Input: part model. Units: mm. Frame: model coordinates. Face numbers are marked on the shaded views. A direction names the side the tool comes from. Coordinates: 2 decimals unless noted, no trailing zeros. Loops run counter-clockwise (first coordinate to the right, second up) from the corner with the lowest first, then second, coordinate; pieces in that order, holes last.
```python
from build123d import *

# Parameters (mm, degrees)
CROQUIS1_W              = 30
CROQUIS1_H              = 30
SALIENTE_EXTRUIR1_DEPTH = 3
CROQUIS2_W              = 3
CROQUIS2_H              = 30
SALIENTE_EXTRUIR2_DEPTH = 30
REDONDEO1_R             = 15
CROQUIS3_R              = 4
CORTAR_EXTRUIR1_DEPTH   = 48.053161424
CROQUIS4_R              = 3
CORTAR_EXTRUIR2_DEPTH   = 37.742346142
CHAFL_N1_SIZE           = 2


with BuildPart() as part:
    # Croquis1 → Saliente-Extruir1 (new body)
    with BuildSketch(Plane(origin=(0, 0, 0), x_dir=(1, 0, 0), z_dir=(0, 1, 0))):
        Rectangle(CROQUIS1_W, CROQUIS1_H)
    extrude(amount=SALIENTE_EXTRUIR1_DEPTH)

    # Croquis2 → Saliente-Extruir2 (add)
    with BuildSketch(Plane(origin=(0, 3, 0), x_dir=(1, 0, 0), z_dir=(0, 1, 0))):
        with Locations((-13.5, 0)):
            Rectangle(CROQUIS2_W, CROQUIS2_H)
        with Locations((13.5, 0)):
            Rectangle(CROQUIS2_W, CROQUIS2_H)
    extrude(amount=SALIENTE_EXTRUIR2_DEPTH)

    # Redondeo1
    redondeo1_edges = [part.edges().sort_by_distance(p)[0] for p in [
        (-13.5, 33, -15),
        (13.5, 33, -15),
        (13.5, 33, 15),
        (-13.5, 33, 15),
    ]]
    fillet(redondeo1_edges, radius=REDONDEO1_R - 0.0001)  # a hair under: the kernel refuses the full size

    # Croquis3 → Cortar-Extruir1 (cut, through all)
    with BuildSketch(Plane(origin=(15, 0, 0), x_dir=(0, 0, -1), z_dir=(1, 0, 0))):
        with Locations((0, 18)):
            Circle(CROQUIS3_R)
    extrude(amount=-CORTAR_EXTRUIR1_DEPTH, mode=Mode.SUBTRACT)

    # Croquis4 → Cortar-Extruir2 (cut, through all)
    with BuildSketch(Plane(origin=(0, 3, 0), x_dir=(1, 0, 0), z_dir=(0, 1, 0))):
        with Locations(Location((0, 0, 0), (0, 0, 270))):
            Circle(CROQUIS4_R)
    extrude(amount=-CORTAR_EXTRUIR2_DEPTH, mode=Mode.SUBTRACT)

    # Chaflán1
    chafl_n1_edges = [part.edges().sort_by_distance(p)[0] for p in [
        (0, 3, -3),
    ]]
    chamfer(chafl_n1_edges, length=CHAFL_N1_SIZE)


solid = part.part
```
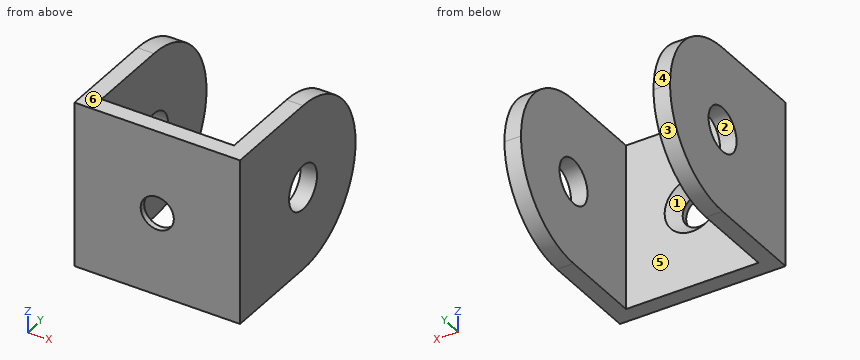
Item 1: Section query B-B (y = 12.5). Output: boundary loops of the cut face in (x, z), then the cut area to 3 significant figures.
Result:
outline: (-15, -15) - (-12, -15) - (-12, 15) - (-15, 15) - close; (12, -15) - (15, -15) - (15, 15) - (12, 15) - close
area: 180 mm2
Item 2: Mould query, pull axis Z, two halves, no side actions, for the marked faces 1, 2, 3 and 4. Classes: +Z half, -Z half, draft (parallel to the pull), parting line (faces both ways), or undercut.
Result:
face 1: undercut
face 2: undercut
face 3: -Z half
face 4: +Z half
Item 3: Section query A-A (x = 0). Output: boundary loops of the cut face in (y, z), then the cut area to 3 significant figures.
Result:
outline: (0, -15) - (3, -15) - (3, -5) - (1, -3) - (0, -3) - close; (0, 3) - (1, 3) - (3, 5) - (3, 15) - (0, 15) - close
area: 68.0 mm2
Item 4: Section query D-D (y = 24.5). Output: boundary loops of the cut face in (x, z).
Result:
outline: (-15, -13.52) - (-12, -13.52) - (-12, 13.52) - (-15, 13.52) - close; (12, -13.52) - (15, -13.52) - (15, 13.52) - (12, 13.52) - close
Item 5: Line query: L1, parallel to Y at x = -14.25, z = 0; L2, parallel to X at y = 23.5, z = -11; L3, parallel to X at y = 0.25, z = 0. Output: solid intervals per line, ascending.
Result:
L1: y = 0 to 14, 22 to 33
L2: x = -15 to -12, 12 to 15
L3: x = -15 to -3, 3 to 15
Item 6: Section query C-C (x = -10). Output: boundary loops of the cut face in (y, z), then the cut area to 3 significant figures.
Result:
outline: (0, -15) - (3, -15) - (3, 15) - (0, 15) - close
area: 90.0 mm2
Item 7: Contact query for flat-ended pins moving along their axis: P1, Ø4, axis at x = -2, z = 6.5, coming from the +Y side; P2, Ø3, axis at x = 12, y = 25, coming from the -Z side; P3, Ø7, axis at x = 0, z = 0, coming from the +Y side. Output: stop coordinate, or through.
Result:
P1: stops at y = 3
P2: stops at z = -13.96
P3: stops at y = 1.5
Item 8: Reachability of the marked faces 5 and 6 from +Z, -Z, +X, -X, +Y, -Y: full face, straight path, thin tool, end or side. Return the list, or none.
Result:
face 5: +Z, -Z, +Y
face 6: +Z, +X, -X, +Y, -Y
